The figure shows three views and two pictorial views of one solid part (mm, origin at its lowest corner). Answer the questions. Give positions to 0.01 mm unless a question says otherwise; leave off trailing zeros. Loops run counter-clockwise (first coordinate to the right, second up) from the corner with the lowest first, then second, coordinate; pieces in that order, holes last.
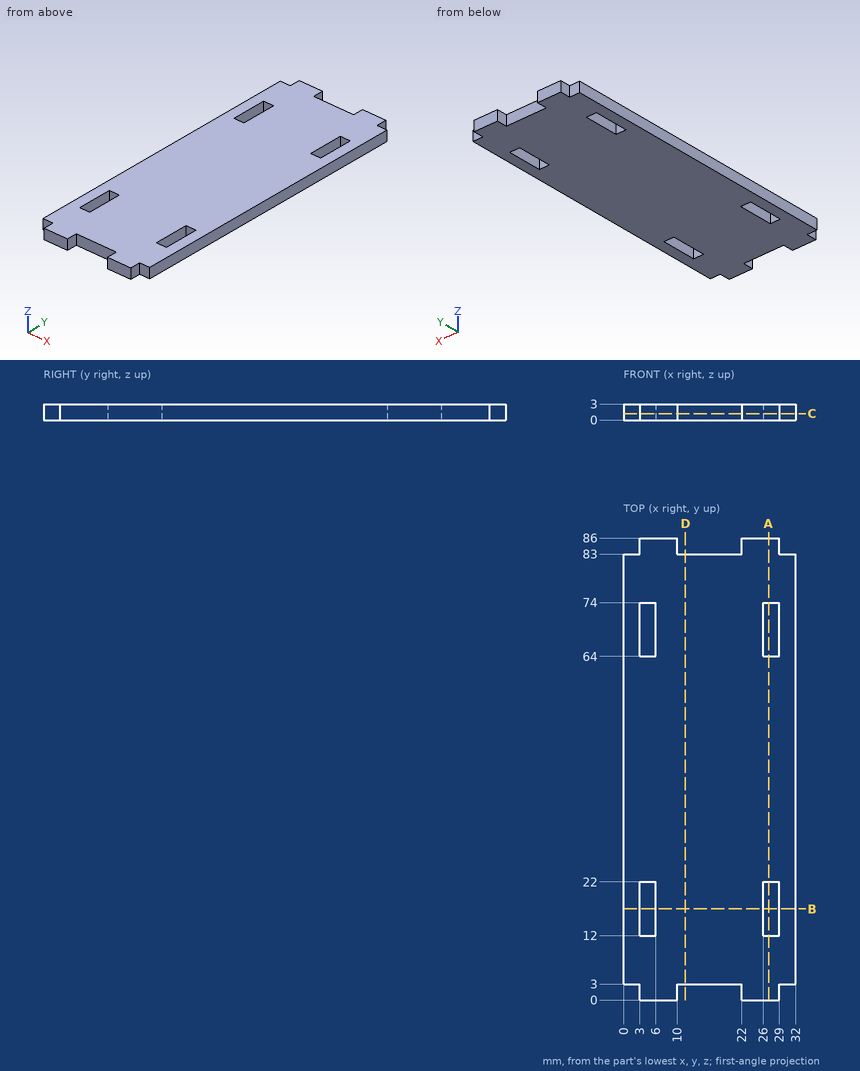
Q1. Consider line 1 along Y through (x, z) = (5.5, 2.75); line 2 along X through (y, z) = (12.5, 0.65); line 3 along Y through (x, z) = (11.5, 2.8). Determine where each line is inside the solid, lowest interval first.
Q2. Section C-C on z = 1.2 is taken. State how many separate pieces and enclosed holes the cut face has, plus the area to 3 significant figures.
Q3. Given pin 1 (1.5 mm diameter, centred on y = 1, z = 1, fed in from -X); pin 2 (1 mm diameter, centred on x = 12, z = 2, fed in from -Y), each flat-ended and moving along its own axis, determine where each tip first touches the part or whether it passes through.
Q4. Section D-D on x = 11.5 is taken. Give the vertices of the cut face in (y, z), plus the area to 3 significant figures.
Q5. Section A-A on x = 27 is taken. Give the vertices of the cut face in (y, z), plus the area to 3 significant figures.
Q6. Section B-B on y = 17 is taken. Give the vertices of the cut face in (x, z), plus the area to 3 significant figures.
Check result:
1. line 1: y = 0 to 12, 22 to 64, 74 to 86
1. line 2: x = 0 to 3, 6 to 26, 29 to 32
1. line 3: y = 3 to 83
2. separate pieces: 1
2. enclosed holes: 4
2. area: 2,520 mm2
3. pin 1: stops at x = 3
3. pin 2: stops at y = 3
4. outline: (3, 0) - (83, 0) - (83, 3) - (3, 3) - close
4. area: 240 mm2
5. outline: (0, 0) - (12, 0) - (12, 3) - (0, 3) - close; (22, 0) - (64, 0) - (64, 3) - (22, 3) - close; (74, 0) - (86, 0) - (86, 3) - (74, 3) - close
5. area: 198 mm2
6. outline: (0, 0) - (3, 0) - (3, 3) - (0, 3) - close; (6, 0) - (26, 0) - (26, 3) - (6, 3) - close; (29, 0) - (32, 0) - (32, 3) - (29, 3) - close
6. area: 78.0 mm2
